Source: CAD feature listing. Evaluate the final solid. Frame: model axes, mm. Face numbers are marked on the shaded views. Give positions to 0.01 mm unless a question says otherwise; leave off trailing zeros. Order: outer loops, then holes, each group sorted by start corner. A loop starts at its lowest first (then second) coordinate and runs counter-clockwise, first axis right, second up. Notation, with made-up numbers: (56.5, 57) - (95.5, 57) arc R29 cw to (95.5, 87) - close; hole circle Ø10 at (31.25, 39). An arc over 180 degrees is marked (long way). Answer as CSV lines item,"result".
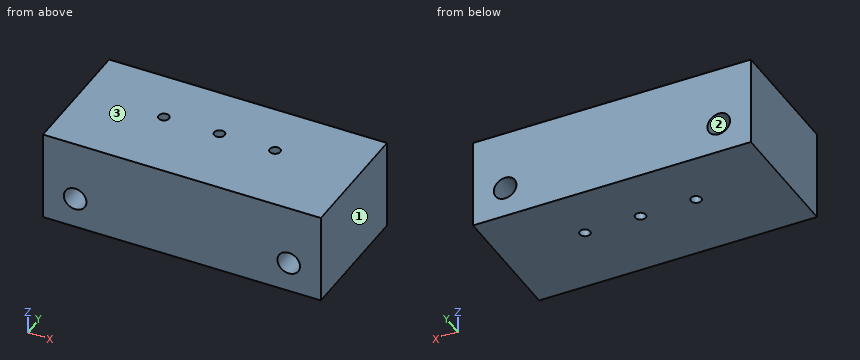
```python
from build123d import *

# Parameters (mm, degrees)
SKETCH_W        = 80
SKETCH_H        = 26
PAD_DEPTH       = 37
SKETCH001_R     = 3.25
POCKET_DEPTH    = 37.501
SKETCH002_R     = 1.5
POCKET001_DEPTH = 26.001


with BuildPart() as part:
    # Sketch → Pad (new body)
    with BuildSketch(Plane.XZ):
        with Locations((0, 13)):
            Rectangle(SKETCH_W, SKETCH_H)
    extrude(amount=PAD_DEPTH)

    # Sketch001 → Pocket (cut, through all)
    with BuildSketch(Plane.XZ.offset(37.5)):
        with Locations((-30.75, 8.75)):
            Circle(SKETCH001_R)
        with Locations((30.75, 8.75)):
            Circle(SKETCH001_R)
    extrude(amount=-POCKET_DEPTH, mode=Mode.SUBTRACT)

    # Sketch002 (on Face6 of Pocket) → Pocket001 (cut, through all)
    with BuildSketch(Plane(origin=(0, 0, 26), x_dir=(-1, 0, 0), z_dir=(0, 0, 1))):
        with Locations((-16, 16)):
            Circle(SKETCH002_R)
        with Locations((16, 16)):
            Circle(SKETCH002_R)
        with Locations((0, 16)):
            Circle(SKETCH002_R)
    extrude(amount=-POCKET001_DEPTH, mode=Mode.SUBTRACT)


solid = part.part
```
(1) Contact query for a flat-ended pin moving along its axis: pin 1 (4 mm diameter, centred on x = -30.75, z = 8.75, fed in from -Y). Output: stop coordinate, or through.
Completed:
pin 1,"through"
(2) Cut plane B-B (z = 8.75). Return loops of the section in (x, y), then the cut area to 3 significant figures.
Completed:
outline,"(-40, -37) - (-34, -37) - (-34, 0) - (-40, 0) - close; (-27.5, -37) - (27.5, -37) - (27.5, 0) - (-27.5, 0) - close; (34, -37) - (40, -37) - (40, 0) - (34, 0) - close; hole circle Ø3 at (-16, -16); hole circle Ø3 at (0, -16); hole circle Ø3 at (16, -16)"
area,"2,460 mm²"
(3) Mould query, pull axis X, two halves, no side actions, for the marked faces 1, 2 and 3. Classes: released by +X, released by -X, zero draft, split by the parting line, or undercut.
Completed:
face 1,"released by +X"
face 2,"undercut"
face 3,"zero draft"
(4) Cut plane D-D (x = 16). Return loops of the section in (y, z), then the cut area to 3 significant figures.
Completed:
outline,"(-37, 0) - (-17.5, 0) - (-17.5, 26) - (-37, 26) - close; (-14.5, 0) - (0, 0) - (0, 26) - (-14.5, 26) - close"
area,"884 mm²"
(5) Cut plane A-A (x = -30.75). Return loops of the section in (y, z), then the cut area to 4 significant figures.
Completed:
outline,"(-37, 0) - (0, 0) - (0, 5.5) - (-37, 5.5) - close; (-37, 12) - (0, 12) - (0, 26) - (-37, 26) - close"
area,"721.5 mm²"
(6) Ray query, line 1 (X direction, y = -16, z = 17); line 2 (Y direction, x = 16, z = 19.5); line 3 (X direction, y = -15, z = 6.75). Return the intervals inside material, ascending. Write a range as from..to.
Completed:
line 1,"-40..-17.5, -14.5..-1.5, 1.5..14.5, 17.5..40"
line 2,"-37..-17.5, -14.5..0"
line 3,"-40..-33.31, -28.19..-17.12, -14.88..-1.12, 1.12..14.88, 17.12..28.19, 33.31..40"
(7) Cut plane C-C (y = -25.5). Return loops of the section in (x, z), then the cut area to 3 significant figures.
Completed:
outline,"(-40, 0) - (40, 0) - (40, 26) - (-40, 26) - close; hole circle Ø6.5 at (-30.75, 8.75); hole circle Ø6.5 at (30.75, 8.75)"
area,"2,010 mm²"
